```python
from build123d import *

# Parameters (mm, degrees)
F0_W      = 234.188
F0_H      = 293.116
F1_DEPTH  = 39.6875
F2_R      = 19.05
F3_R      = 19.05
F4_R      = 19.05
F5_R      = 19.05
F6_R      = 6.35
F7_DEPTH  = 31.75
F8_R      = 4.7625
F9_DEPTH  = 31.75
F10_W     = 12.7
F10_H     = 15.875
F11_DEPTH = 31.75


with BuildPart() as f1:
    # F0 (on Front) → F1 (new body)
    with BuildSketch(Plane.XZ):
        with Locations((0.527771, -8.937072)):
            Rectangle(F0_W, F0_H)
    extrude(amount=F1_DEPTH)

    # F2
    f2_edges = [f1.edges().sort_by_distance(p)[0] for p in [
        (117.621771, -19.84375, 137.620928),
    ]]
    fillet(f2_edges, radius=F2_R)

    # F3
    f3_edges = [f1.edges().sort_by_distance(p)[0] for p in [
        (-116.566229, -19.84375, 137.620928),
    ]]
    fillet(f3_edges, radius=F3_R)

    # F4
    f4_edges = [f1.edges().sort_by_distance(p)[0] for p in [
        (-116.566229, -19.84375, -155.495072),
    ]]
    fillet(f4_edges, radius=F4_R)

    # F5
    f5_edges = [f1.edges().sort_by_distance(p)[0] for p in [
        (117.621771, -19.84375, -155.495072),
    ]]
    fillet(f5_edges, radius=F5_R)

    # F6 (on face) → F7 (join)
    with BuildSketch(Plane.YZ.offset(117.621771)):
        with Locations((-19.84375, -104.695072)):
            Circle(F6_R)
    extrude(amount=F7_DEPTH)

    # F8 (on face) → F9 (join)
    with BuildSketch(Plane.YZ.offset(117.621771)):
        with Locations((-19.84375, -120.570072)):
            Circle(F8_R)
    extrude(amount=F9_DEPTH)

    # F10 (on face) → F11 (join)
    with BuildSketch(Plane.YZ.offset(117.621771)):
        with Locations((-19.84375, 9.033428)):
            Rectangle(F10_W, F10_H)
    extrude(amount=F11_DEPTH)


solid = f1.part
```
Model file for the job. Use its own axes, mm. A direction names the side the tool comes from. Give positions to 0.01 mm unless a question says otherwise; leave off trailing zeros. Order: outer loops, then holes, each group sorted by start corner. A loop starts at its lowest first (then second) coordinate and runs counter-clockwise, first axis right, second up.
1) 3-axis set-ups, long thin cutter, end or side, ignore diameter. For faces 1 (the flat face through (133, -26.194, 9)), 2 (the cylindrical face through (133.27, -16.43, -99.34)), 3 (the flat face through (133, -20, 16.971)): which of +Z, -Z, +X, -X, +Y, -Y reach the whole face in a straight line?
2) Saw through at A-A, the plane y = -20.5. Write the cut outline in (x, z), then the cut area to 3 significant figures.
3) Mould opens along Z. For faces 4 (the flat face through (133, -20, 1.096)), 5 (the flat face through (133, -13.494, 9)), 6 (the cylindrical face through (133.27, -20.88, -125.22)), 7 (the cylindrical face through (-111.1, -20.1, -149.8)) say: +Z half, -Z half, draft (parallel to the pull), parting line (faces both ways), or undercut.
4) Saw through at B-B, the plane z = 90. Write the cut outline in (x, y).
5) Wall check: probe 1 along X at (y, z) = (-12, -49); probe 2 along Z at (x, y) = (125, -18); probe 3 along Z at (x, y) = (-101, -28). Give the ranges that are in metal, low to high.
6) Pin check, flat tips, straight feed: pin 1 (8 mm diameter, centred on x = 138, z = 10, fed in from +Y); pin 2 (12 mm diameter, centred on y = -16, z = 79.5, fed in from +X); pin 3 (5 mm diameter, centred on x = 139, z = 9.5, fed in from -Y). Stop position of each tip, or through.
Computed:
1. face 1: +Z, -Z, +X, -Y
1. face 2: +X
1. face 3: +Z, +X, +Y, -Y
2. outline: (-116.57, -136.45) arc R19.05 ccw to (-97.52, -155.5) - (98.57, -155.5) arc R19.05 ccw to (117.62, -136.45) - (117.62, -125.29) - (149.37, -125.29) - (149.37, -115.85) - (117.62, -115.85) - (117.62, -111.01) - (149.37, -111.01) - (149.37, -98.38) - (117.62, -98.38) - (117.62, 1.1) - (149.37, 1.1) - (149.37, 16.97) - (117.62, 16.97) - (117.62, 118.57) arc R19.05 ccw to (98.57, 137.62) - (-97.52, 137.62) arc R19.05 ccw to (-116.57, 118.57) - close
2. area: 69,500 mm2
3. face 4: undercut
3. face 5: draft
3. face 6: undercut
3. face 7: -Z half
4. outline: (-116.57, -39.69) - (117.62, -39.69) - (117.62, 0) - (-116.57, 0) - close
5. probe 1: x = -116.57 to 117.62
5. probe 2: z = -124.96 to -116.18, -110.77 to -98.62, 1.1 to 16.97
5. probe 3: z = -155.17 to 137.3
6. pin 1: stops at y = -13.49
6. pin 2: stops at x = 117.62
6. pin 3: stops at y = -26.19
